from build123d import *

# Parameters (mm, degrees)
F1_DEPTH = 6
F2_R     = 5


with BuildPart() as f1:
    # F0 (on Top) → F1 (new body)
    with BuildSketch(Plane.XY):
        with BuildLine():
            Line((195, -175), (225, -175))
            Line((225, -175), (225, 175))
            ThreePointArc((225, 175), (29.4969127553, 131.3574891295), (-153.5716205835, 50.0430501997))
            ThreePointArc((-153.5716205835, 50.0430501997), (-205.8843017039, -2.9969136264), (-225, -75))
            Line((-225, -75), (195, -175))
        make_face()
    extrude(amount=F1_DEPTH)

    # F2
    f2_edges = [f1.edges().sort_by_distance(p)[0] for p in [
        (225, 175, 3),
        (195, -175, 3),
    ]]
    fillet(f2_edges, radius=F2_R)


solid = f1.part
Model file for the job. Use its own axes, mm. Round coordinates to 2 decimals unless told otherwise and drop trailing zeros. Order: outer loops, then holes, each group sorted by start corner. A loop starts at its lowest first (then second) coordinate and runs counter-clockwise, first axis right, second up.
(1) Pin check, flat tips, straight feed: pin 1 (1 mm diameter, centred on x = 56.5, z = 3.5, fed in from +Y); pin 2 (1 mm diameter, centred on y = 58.5, z = 2, fed in from -X). Stop position of each tip, or through.
(2) Band-saw the part on A-A (z = 3.8). List the corners of the cut face in (x, y), then the cut area to 3 significant figures.
(3) Band-saw the part on B-B (y = -116). List the corners of the cut face in (x, z), then the cut area to 3 significant figures.
(4) Drill centre lines: line 1 (X direction, y = -72.5, z = 5.5); line 2 (Y direction, x = -61, z = 0.7); line 3 (X direction, y = -22.5, z = 0.5). Where is each one in solid material? Low to high.
(5) Band-saw the part on C-C (x = 163). List the corners of the cut face in (y, z), then the cut area to 3 significant figures.
Verdict:
1. pin 1: stops at y = 140
1. pin 2: stops at x = -139.32
2. outline: (-225, -75) - (194.43, -174.86) arc R5 ccw to (195.59, -175) - (225, -175) - (225, 169.34) arc R5 ccw to (219.37, 174.3) arc R1011.47 ccw to (-153.57, 50.04) arc R145.16 ccw to start
2. area: 107,000 mm2
3. outline: (-52.8, 0) - (225, 0) - (225, 6) - (-52.8, 6) - close
3. area: 1,670 mm2
4. line 1: x = -224.98 to 225
4. line 2: y = -114.05 to 96.59
4. line 3: x = -215.17 to 225
5. outline: (-167.38, 0) - (165.54, 0) - (165.54, 6) - (-167.38, 6) - close
5. area: 2,000 mm2
